Could you check a few things on this drawing? It's one solid part, dimensions in mm from its lowest x, y, z. Give positions to 0.01 mm unless a question says otherwise; leave off trailing zeros. Order: outer loops, then holes, each group sorted by start corner. A loop starts at its lowest first (then second) coordinate and runs counter-clockwise, first axis right, second up. Notation, with made-up numbers: (35, 24) -> (76, 24) arc R14 ccw to (76, 46) -> close; hole circle Ø6 at (24, -23). An arc over 180 degrees is marked (long way). Answer as CSV lines item,"result".
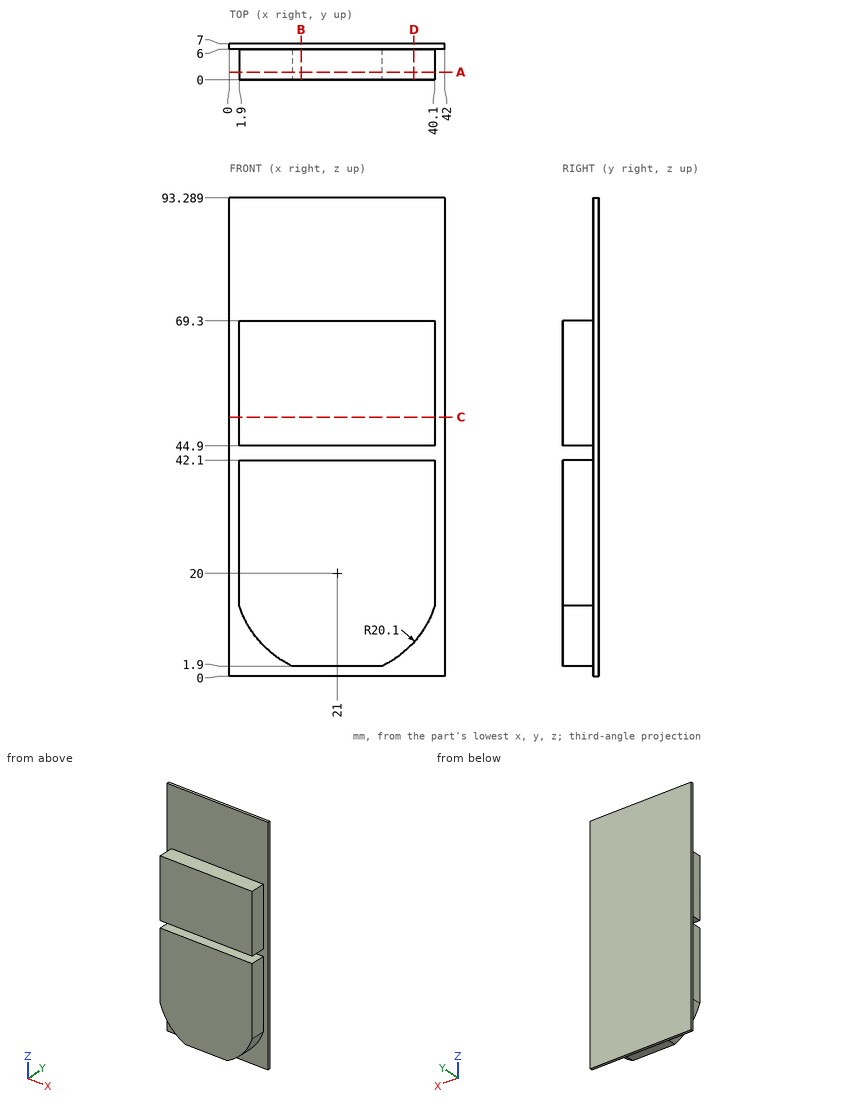
Item 1: Please list where these lines run through material, in increasing order: line 1 along Z through (x, y) = (14, 3); line 2 along Y through (x, z) = (32.5, 77); line 3 along X through (y, z) = (5.75, 51).
Numbers:
line 1,"z = 1.9 to 42.1, 44.9 to 69.3"
line 2,"y = 6 to 7"
line 3,"x = 1.9 to 40.1"
Item 2: Imagine slicing it at A-A, the plane y = 1.5. Please give me the cut outline in (x, z).
Numbers:
outline,"(1.9, 13.74) arc R20.1 ccw to (12.26, 1.9) -> (29.74, 1.9) arc R20.1 ccw to (40.1, 13.74) -> (40.1, 42.1) -> (1.9, 42.1) -> close; (1.9, 44.9) -> (40.1, 44.9) -> (40.1, 69.3) -> (1.9, 69.3) -> close"
Item 3: Imagine slicing it at C-C, the plane z = 50.5. Please give me the cut outline in (x, y), then the cut area to 3 significant figures.
Numbers:
outline,"(0, 6) -> (1.9, 6) -> (1.9, 0) -> (40.1, 0) -> (40.1, 6) -> (42, 6) -> (42, 7) -> (0, 7) -> close"
area,"271 mm²"
Item 4: Imagine slicing it at B-B, the plane x = 14. Please give me the cut outline in (y, z).
Numbers:
outline,"(0, 1.9) -> (6, 1.9) -> (6, 0) -> (7, 0) -> (7, 93.29) -> (6, 93.29) -> (6, 69.3) -> (0, 69.3) -> (0, 44.9) -> (6, 44.9) -> (6, 42.1) -> (0, 42.1) -> close"
Item 5: Imagine slicing it at D-D, the plane x = 36. Please give me the cut outline in (y, z).
Numbers:
outline,"(0, 6.62) -> (6, 6.62) -> (6, 0) -> (7, 0) -> (7, 93.29) -> (6, 93.29) -> (6, 69.3) -> (0, 69.3) -> (0, 44.9) -> (6, 44.9) -> (6, 42.1) -> (0, 42.1) -> close"
Item 6: For pin 1 (1 mm diameter, centred on y = 1.5, z = 68, fed in from +X); pin 2 (1.5 mm diameter, centred on y = 5, z = 16.5, fed in from -X); pin 3 (4 mm diameter, centred on x = 35, y = 2, fed in from -Z) (1 decimal), each with a flat end and sliding along its axis, tell me the tip position at first contact or that it passes through.
Numbers:
pin 1,"stops at x = 40.1"
pin 2,"stops at x = 1.9"
pin 3,"stops at z = 3.9"
